Read the model definition and answer for the solid it produces. Units are mm, in the model's axes. Face numbers are marked on the shaded views. A direction names the side the tool comes from. Round coordinates to 2 decimals unless told otherwise and drop trailing zeros. Loops run counter-clockwise (first coordinate to the right, second up) from the corner with the lowest first, then second, coordinate; pieces in that order, holes last. Notation, with made-up numbers: M 39.5,-28.5 L 87.5,-28.5 A9 cw 87.5,-17.5 Z; hole C 32.25,-9.5 d11. An arc over 180 degrees is marked long. Write each question's results on one line, items separated by ' | '.
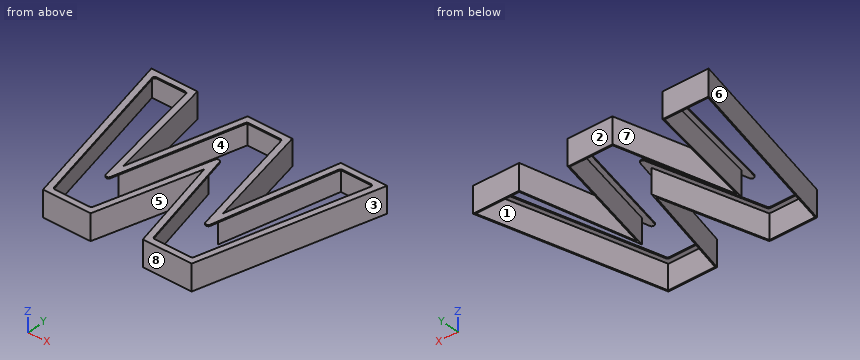
from build123d import *

# Parameters (mm, degrees)
BOSS_EXTRUDE1_DEPTH      = 1
BOSS_EXTRUDE1_DEPTH_BACK = 20
CUT_EXTRUDE1_DEPTH       = 20
CUT_EXTRUDE2_DEPTH       = 213.08892348854144
FILLET1_R                = 2


with BuildPart() as part:
    # Sketch1 → Boss-Extrude1 (new, two sides: drawn at the far end of the back side and taken through both)
    with BuildSketch(Plane.XY.offset(-BOSS_EXTRUDE1_DEPTH_BACK)):
        Polygon((2646.8216415771526, -1645.5825778387778), (2668.443454041995, -1563.4301992512205), (2689.750003141614, -1645.5825778387778), (2729.823511169442, -1645.5825778387778), (2765.5169447137464, -1502.5825778387775), (2727.659454154938, -1502.5825778387775), (2708.6195188972147, -1591.9057308997028), (2687.7252140876417, -1502.5825778387775), (2650.9700988373584, -1502.5825778387775), (2628.472349976695, -1593.6984607244628), (2609.9247872531955, -1502.5825778387775), (2572.055836643681, -1502.5825778387775), (2607.749270187985, -1645.5825778387778), align=None)
    extrude(amount=BOSS_EXTRUDE1_DEPTH + BOSS_EXTRUDE1_DEPTH_BACK)

    # 3DSketch1 → Cut-Extrude1 (cut)
    with BuildSketch(Plane(origin=(2690.52373407352, -1644.582577838785, -20), x_dir=(-0.6391782942740818, 0.7690585856284783, 0), z_dir=(0, 0, -1))):
        Polygon((0, 0), (79.56194930817296, 37.42380228418931), (28.42614813473769, -34.202308612791946), (52.4083937415845, -63.05771883529219), (183.34103881667534, -1.388e-14), (160.4765333052003, 27.510546630372875), (75.35406283201465, -18.178865153681013), (133.21853325786614, 60.30734081323959), (110.73293100318098, 87.3619914825534), (25.390706940818667, 44.69138476980368), (84.18362231643819, 119.30608903866502), (61.32155847684101, 146.81369785225445), (-24.620317595277953, 29.62313770222462), align=None)
    extrude(amount=-CUT_EXTRUDE1_DEPTH, mode=Mode.SUBTRACT)

    # 3DSketch2 → Cut-Extrude2 (cut, through all)
    with BuildSketch(Plane(origin=(2605.8400476167385, -1507.582577838778, 1), x_dir=(0.6701296542123282, -0.7422440613068356, 0), z_dir=(0, 0, 1))):
        Polygon((0, 0), (-18.350017001032523, -20.32471038743184), (102.61499812527803, -84.81138938300774), (123.59854919676319, -61.56974342682699), (68.74754201218234, 22.323071235087976), (157.54150984392544, -23.97409189109885), (179.1863444024586, 0), (102.71443922113765, 113.76780902490334), (84.34650287386148, 93.42325094344824), (148.62854454728856, 4.588347978661769), (52.21635833956266, 57.83549741007506), (32.86694064083099, 36.40383819852962), (95.66426345437596, -56.51066473506117), align=None)
    extrude(amount=-CUT_EXTRUDE2_DEPTH, mode=Mode.SUBTRACT)

    # Fillet1
    fillet1_edges = [part.edges().sort_by_distance(p)[0] for p in [
        (2611.6546507267108, -1640.5825778387798, 0.5),
        (2642.967324236363, -1640.5825778387775, 0.5),
        (2578.4572614861936, -1507.5825778387775, 0.5),
        (2605.8400476167385, -1507.582577838778, 0.5),
        (2654.885691895029, -1507.5825778387768, 0.5),
        (2683.7598322604117, -1507.5825778387764, 0.5),
        (2668.478981227683, -1543.650680619036, 0.5),
        (2693.618657801144, -1640.5825778387807, 0.5),
        (2725.918130630729, -1640.5825778387841, 0.5),
        (2759.115519871237, -1507.5825778387766, 0.5),
        (2731.7059936223714, -1507.582577838777, 0.5),
        (2708.8461168186655, -1614.826444325335, 0.5),
        (2628.0028021057956, -1616.4582814852965, 0.5),
    ]]
    fillet(fillet1_edges, radius=FILLET1_R)


solid = part.part
Item 1: For the marked faces 4, 5, 6, 7 and 8, determine the directions among +Z, -Z, +X, -X, +Y, -Y from which every point of the face is accessible in a straight line to the end or side of a thin tool.
Outcome:
face 4: -Z | face 5: +Z, -Z, -Y | face 6: +Z, -Z, -X, -Y | face 7: +Z, -Z, +Y | face 8: +Z, -Z, +X, -X, -Y
Item 2: The part is cut by section B-B (x = 2740.5). Determine the outline of the cut face in (y, z), plus the area to 3 significant figures.
Outcome:
outline: M -1602.81,-20 L -1598.68,-20 L -1598.68,0 L -1582.16,0 L -1582.16,1 L -1602.81,1 Z; M -1507.58,0 L -1503.58,0 L -1503.58,-20 L -1502.58,-20 L -1502.58,1 L -1507.58,1 Z | area: 128 mm2
Item 3: Flat-ended cylindrical pins translate along their axes: pin 1 (2 mm diameter, centred on y = -1611, z = -15.5, fed in from +X); pin 2 (4 mm diameter, centred on y = -1520, z = -11.5, fed in from +X); pin 3 (6 mm diameter, centred on y = -1542, z = -1.5, fed in from +X). Find the tip coordinate at first contact, or state that the pin passes through.
Outcome:
pin 1: stops at x = 2738.71 | pin 2: stops at x = 2761.67 | pin 3: stops at x = 2756.43
Item 4: The part is cut by section A-A (z = -12). Determine the outline of the cut face in (x, y), plus the area to 3 significant figures.
Outcome:
outline: M 2572.06,-1502.58 L 2607.75,-1645.58 L 2646.82,-1645.58 L 2668.44,-1563.43 L 2689.75,-1645.58 L 2729.82,-1645.58 L 2765.52,-1502.58 L 2727.66,-1502.58 L 2708.62,-1591.91 L 2687.73,-1502.58 L 2650.97,-1502.58 L 2628.47,-1593.7 L 2609.92,-1502.58 Z; hole M 2573.34,-1503.58 L 2608.53,-1644.58 L 2646.05,-1644.58 L 2668.45,-1559.47 L 2690.52,-1644.58 L 2729.04,-1644.58 L 2764.24,-1503.58 L 2728.47,-1503.58 L 2708.66,-1596.49 L 2686.93,-1503.58 L 2651.75,-1503.58 L 2628.38,-1598.25 L 2609.11,-1503.58 Z | area: 1,030 mm2
Item 5: Straight lines are drawn through the part: line 1 (X direction, y = -1602, z = -18.75); line 2 (X direction, y = -1549.5, z = -0.75); line 3 (X direction, y = -1622, z = -7.5). For each, find the intervals that lie inside material, in ascending order.
Outcome:
line 1: x = 2596.87 to 2597.9, 2657.26 to 2658.29, 2678.45 to 2679.48, 2739.67 to 2740.7 | line 2: x = 2583.77 to 2584.8, 2618.45 to 2619.48, 2639.39 to 2640.42, 2697.67 to 2698.7, 2717.66 to 2718.68, 2752.78 to 2753.81 | line 3: x = 2601.86 to 2602.89, 2651.99 to 2653.03, 2683.63 to 2684.67, 2734.68 to 2735.71
Item 6: The part is cut by section D-D (y = -1531.5). State how many separate pieces and enclosed holes the cut face has, plus the area to 3 significant figures.
Outcome:
separate pieces: 6 | enclosed holes: 0 | area: 154 mm2
Item 7: The mould has two halves that part along Y. Classify the marked faces 1, 2 and 3: pulls with the +Y half, pulls with the -Y half, needs draft (parallel to the pull), parting line crosses it, or undercut.
Outcome:
face 1: undercut | face 2: pulls with the +Y half | face 3: pulls with the -Y half
Item 8: The part is cut by section C-C (y = -1623). Determine the outline of the cut face in (x, z).
Outcome:
outline: M 2602.11,-20 L 2603.14,-20 L 2603.14,0 L 2607.27,0 L 2607.27,1 L 2602.11,1 Z; M 2647.59,0 L 2651.73,0 L 2651.73,-20 L 2652.77,-20 L 2652.77,1 L 2647.59,1 Z; M 2683.89,-20 L 2684.93,-20 L 2684.93,0 L 2689.06,0 L 2689.06,1 L 2683.89,1 Z; M 2730.31,0 L 2734.43,0 L 2734.43,-20 L 2735.46,-20 L 2735.46,1 L 2730.31,1 Z
